from build123d import *

# Parameters (mm, degrees)
BOSS_EXTRUDE1_DEPTH = 40
SKETCH4_W           = 11.8
SKETCH4_H           = 32.3
CUT_EXTRUDE1_DEPTH  = 5.5
SKETCH5_W           = 11.8
SKETCH5_H           = 22.5
CUT_EXTRUDE2_DEPTH  = 9.498848241
SKETCH6_R           = 1.25
CUT_EXTRUDE3_DEPTH  = 9.498848241
SKETCH7_W           = 12
SKETCH7_H           = 13.998848241
BOSS_EXTRUDE2_DEPTH = 10
SKETCH8_W           = 8
SKETCH8_H           = 9.998848241
CUT_EXTRUDE6_DEPTH  = 10
SKETCH9_R           = 2
CUT_EXTRUDE7_DEPTH  = 14.998848241


with BuildPart() as part:
    # Sketch1 → Boss-Extrude1 (new body)
    with BuildSketch(Plane.XY):
        Polygon((8.670952565, 9.003587153), (-11.329047435, 9.003587153), (-21.329047435, 9.003587153), (-21.329047435, -4.995261088), (-11.329047435, -4.995261088), (8.670952565, -4.995261088), align=None)
    extrude(amount=BOSS_EXTRUDE1_DEPTH)

    # Sketch4 → Cut-Extrude1 (cut)
    with BuildSketch(Plane(origin=(0, 9.003587153, 0), x_dir=(1, 0, 0), z_dir=(0, 1, 0))):
        with Locations((-6.329047435, -20)):
            Rectangle(SKETCH4_W, SKETCH4_H)
    extrude(amount=-CUT_EXTRUDE1_DEPTH, mode=Mode.SUBTRACT)

    # Sketch5 → Cut-Extrude2 (cut, through all)
    with BuildSketch(Plane(origin=(0, 3.503587153, 0), x_dir=(1, 0, 0), z_dir=(0, 1, 0))):
        with Locations((-6.329047435, -20)):
            Rectangle(SKETCH5_W, SKETCH5_H)
    extrude(amount=-CUT_EXTRUDE2_DEPTH, mode=Mode.SUBTRACT)

    # Sketch6 → Cut-Extrude3 (cut, through all)
    with BuildSketch(Plane(origin=(0, 3.503587153, 0), x_dir=(1, 0, 0), z_dir=(0, 1, 0))):
        with Locations((-6.329047435, -6.3)):
            Circle(SKETCH6_R)
        with Locations((-6.329047435, -33.7)):
            Circle(SKETCH6_R)
    extrude(amount=-CUT_EXTRUDE3_DEPTH, mode=Mode.SUBTRACT)

    # Sketch7 → Boss-Extrude2 (add)
    with BuildSketch(Plane.ZY.offset(21.329047435)):
        with Locations((6, 2.004163032)):
            Rectangle(SKETCH7_W, SKETCH7_H)
    extrude(amount=BOSS_EXTRUDE2_DEPTH)

    # Sketch8 → Cut-Extrude6 (cut)
    with BuildSketch(Plane.ZY.offset(31.329047435)):
        with Locations((6, 2.004163033)):
            Rectangle(SKETCH8_W, SKETCH8_H)
    extrude(amount=-CUT_EXTRUDE6_DEPTH, mode=Mode.SUBTRACT)

    # Sketch9 → Cut-Extrude7 (cut, through all)
    with BuildSketch(Plane(origin=(0, 9.003587153, 0), x_dir=(1, 0, 0), z_dir=(0, 1, 0))):
        with Locations((-26.329047435, -6)):
            Circle(SKETCH9_R)
    extrude(amount=-CUT_EXTRUDE7_DEPTH, mode=Mode.SUBTRACT)


solid = part.part
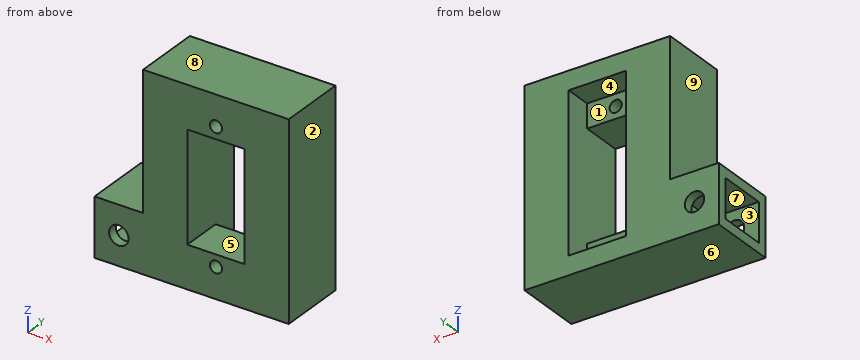
Here's how the part is built. I have some questions about the finished solid (model axes, mm). Face numbers are marked on the shaded views. A direction names the side the tool comes from. Give positions to 0.01 mm unless a question says otherwise; leave off trailing zeros. Loops run counter-clockwise (first coordinate to the right, second up) from the corner with the lowest first, then second, coordinate; pieces in that order, holes last. Notation, with made-up numbers: (-30.5, 38.25) -> (24.5, 38.25) arc R18 cw to (24.5, 46.25) -> close; hole circle Ø11 at (-10, -12). An arc over 180 degrees is marked (long way). Answer as a JSON object with one key per item and string values. Group by question number.
Item 1: Imagine slicing it at A-A on y = 8. Write out the boundary of the cut face in (x, z).
Item 2: Imagine slicing it at D-D on y = 4.5. Write out the boundary of the cut face in (x, z).
Item 3: Imagine slicing it at B-B on z = 16. Write out the boundary of the cut face in (x, y).
Item 4: I need wall thicknesses on L1, parallel to X at y = 4.75, z = 16.5; L2, parallel to X at y = -0.75, z = 6.3; L3, parallel to X at y = -4.4, z = 6. Which ranges of each line are inside material? Lowest first, please.
Item 5: On a 3-axis mill with a long thin cutter (end or side, diameter ignored), from which of +Z, -Z, +X, -X, +Y, -Y can I reach the whole of each face in a straight line? I mean the marked faces 5, 6, 7, 8 and 9. Say none if no direction works.
Item 6: Will these pins go through, and if not, where does the flat tip stop? pin 1 (4 mm diameter, centred on y = 1.5, z = 32.5, fed in from -X); pin 2 (1.5 mm diameter, centred on x = -7, z = 7, fed in from +Y); pin 3 (2 mm diameter, centred on x = -6.33, z = 6.3, fed in from +Y); pin 4 (3 mm diameter, centred on x = -28.5, y = 0, fed in from +Z).
Item 7: Thinking about a two-plate mould opening in X: for the marked faces 1, 2, 3 and 4, which applies, pulls with the +X half, pulls with the -X half, needs draft (parallel to the pull), parting line crosses it, or undercut?
Item 8: Imagine slicing it at C-C on x = -23.5. Write out the boundary of the cut face in (y, z), then the cut area to 3 significant figures.
Answer list:
{
 "1": {"outline": "(-31.33, 0) -> (8.67, 0) -> (8.67, 40) -> (-21.33, 40) -> (-21.33, 12) -> (-31.33, 12) -> close; hole circle Ø4 at (-26.33, 6); hole (-12.23, 3.85) -> (-0.43, 3.85) -> (-0.43, 36.15) -> (-12.23, 36.15) -> close"},
 "2": {"outline": "(-31.33, 0) -> (8.67, 0) -> (8.67, 40) -> (-21.33, 40) -> (-21.33, 12) -> (-31.33, 12) -> (-31.33, 10) -> (-21.33, 10) -> (-21.33, 2) -> (-31.33, 2) -> close; hole (-12.23, 3.85) -> (-0.43, 3.85) -> (-0.43, 36.15) -> (-12.23, 36.15) -> close"},
 "3": {"outline": "(-21.33, -5) -> (-12.23, -5) -> (-12.23, 9) -> (-21.33, 9) -> close; (-0.43, -5) -> (8.67, -5) -> (8.67, 9) -> (-0.43, 9) -> close"},
 "4": {"L1": "x = -21.33 to -12.23, -0.43 to 8.67", "L2": "x = -21.33 to -7.58, -5.08 to 8.67", "L3": "x = -31.33 to -28.33, -24.33 to -7.54, -5.12 to 8.67"},
 "5": {"face 5": "+Y, -Y", "face 6": "-Z, +X, -X, +Y, -Y", "face 7": "-X", "face 8": "+Z, +X, -X, +Y, -Y", "face 9": "+Z, -X, +Y, -Y"},
 "6": {"pin 1": "stops at x = -21.33", "pin 2": "stops at y = 3.5", "pin 3": "passes through", "pin 4": "stops at z = 12"},
 "7": {"face 1": "undercut", "face 2": "pulls with the +X half", "face 3": "needs draft", "face 4": "undercut"},
 "8": {"outline": "(-5, 0) -> (9, 0) -> (9, 12) -> (-5, 12) -> close; hole (-3, 2) -> (7, 2) -> (7, 10) -> (-3, 10) -> close", "area": "88.0 mm2"}
}
